```python
from build123d import *

# Parameters (mm, degrees)
F0_W     = 3.848
F0_H     = 8
F0_R     = 6
F0_R_2   = 4.05
F1_DEPTH = 5
F2_DEPTH = 3
F3_DEPTH = 50
F4_R     = 1


with BuildPart() as f1:
    # F0 (on Top) → F1 (new body)
    with BuildSketch(Plane.XY):
        with BuildLine():
            ThreePointArc((-8.75, 9.683053), (-3.977029, 7.706024), (-2, 2.933053))
            ThreePointArc((-2, 2.933053), (-3.977029, -1.839918), (-8.75, -3.816947))
            Line((-8.75, -3.816947), (8.75, -3.816947))
            ThreePointArc((8.75, -3.816947), (2, 2.933053), (8.75, 9.683053))
            Line((8.75, 9.683053), (-8.75, 9.683053))
        make_face()
        with Locations((0, 2.933053)):
            Rectangle(F0_W, F0_H, mode=Mode.SUBTRACT)
        with BuildLine():
            ThreePointArc((-8.75, -3.816947), (-3.977029, -1.839918), (-2, 2.933053))
            ThreePointArc((-2, 2.933053), (-3.977029, 7.706024), (-8.75, 9.683053))
            ThreePointArc((-8.75, 9.683053), (-15.5, 2.933053), (-8.75, -3.816947))
        make_face()
        with Locations((-8.75, 2.933053)):
            Circle(F0_R, mode=Mode.SUBTRACT)
        with BuildLine():
            ThreePointArc((15.5, 2.933053), (13.522971, 7.706024), (8.75, 9.683053))
            ThreePointArc((8.75, 9.683053), (2, 2.933053), (8.75, -3.816947))
            ThreePointArc((8.75, -3.816947), (13.522971, -1.839918), (15.5, 2.933053))
        make_face()
        with Locations((8.75, 2.933053)):
            Circle(F0_R, mode=Mode.SUBTRACT)
        with Locations((-8.75, 2.933053)):
            Circle(F0_R)
        with Locations((-8.75, 2.933053)):
            Circle(F0_R_2, mode=Mode.SUBTRACT)
        with Locations((8.75, 2.933053)):
            Circle(F0_R)
        with Locations((8.75, 2.933053)):
            Circle(F0_R_2, mode=Mode.SUBTRACT)
    extrude(amount=F1_DEPTH)

    # F0 (on Top) → F2 (cut)
    with BuildSketch(Plane.XY):
        with Locations((-8.75, 2.933053)):
            Circle(F0_R)
        with Locations((-8.75, 2.933053)):
            Circle(F0_R_2, mode=Mode.SUBTRACT)
        with Locations((8.75, 2.933053)):
            Circle(F0_R)
        with Locations((8.75, 2.933053)):
            Circle(F0_R_2, mode=Mode.SUBTRACT)
    extrude(amount=F2_DEPTH, mode=Mode.SUBTRACT)

    # F0 (on Top) → F3 (join)
    with BuildSketch(Plane.XY):
        with Locations((0, 2.933053)):
            Rectangle(F0_W, F0_H)
    extrude(amount=F3_DEPTH)

    # F4
    f4_edges = [f1.edges().sort_by_distance(p)[0] for p in [
        (-1.924, -1.066947, 27.5),
        (1.924, -1.066947, 27.5),
        (1.924, 6.933053, 27.5),
        (-1.924, 6.933053, 27.5),
    ]]
    fillet(f4_edges, radius=F4_R)


solid = f1.part
```
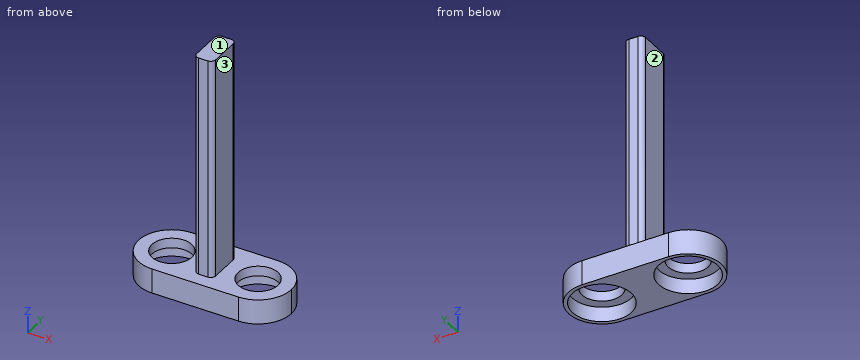
Read the model definition and answer for the solid it produces. Units are mm, in the model's axes. Face numbers are marked on the shaded views. A direction names the side the tool comes from. Give positions to 0.01 mm unless a question says otherwise; leave off trailing zeros. Write each loop counter-clockwise with the first axis right and the second up, starting at its lowest first coordinate (ties: lowest second). Pieces come first, ordered by that corner, then holes. Notation, with made-up numbers: (28, 6) -> (50, 6) arc R12 ccw to (50, 21) -> close; hole circle Ø4 at (42, 47.25). An arc over 180 degrees is marked (long way). Answer as a JSON object with one key per item and string values.
1) Section B-B on x = -6.5 is taken. Write down the section's boundary in (y, z).
Findings below:
{"outline": "(-3.82, 0) -> (-2.63, 0) -> (-2.63, 3) -> (-0.43, 3) -> (-0.43, 5) -> (-3.82, 5) -> close; (6.3, 3) -> (8.5, 3) -> (8.5, 0) -> (9.68, 0) -> (9.68, 5) -> (6.3, 5) -> close"}
2) A tool of negligible diameter and unlimited length cuts with its end or side. For the marked faces 1, 2 and 3, from which of +Z, -Z, +X, -X, +Y, -Y can it reach the whole face along a straight path? Write none if from no direction.
Findings below:
{"face 1": "+Z, +X, -X, +Y, -Y", "face 2": "+Z, -X, +Y, -Y", "face 3": "+Z, +X, +Y, -Y"}
3) Section D-D on y = 0.5 is taken. Write down the section's boundary in (x, z).
Findings below:
{"outline": "(-15.05, 0) -> (-14.23, 0) -> (-14.23, 3) -> (-11.99, 3) -> (-11.99, 5) -> (-15.05, 5) -> close; (-5.51, 3) -> (-3.27, 3) -> (-3.27, 0) -> (3.27, 0) -> (3.27, 3) -> (5.51, 3) -> (5.51, 5) -> (1.92, 5) -> (1.92, 50) -> (-1.92, 50) -> (-1.92, 5) -> (-5.51, 5) -> close; (11.99, 3) -> (14.23, 3) -> (14.23, 0) -> (15.05, 0) -> (15.05, 5) -> (11.99, 5) -> close"}
4) Straight lines are drawn through the part: probe 1 along Y at (x, z) = (-8.75, 0.8); probe 2 along Y at (x, z) = (9, 3.5); probe 3 along Z at (x, y) = (-4, 9). For each, find the intervals that lie inside material, in ascending order. Write a range as from..to.
Findings below:
{"probe 1": "y = -3.82..-3.07, 8.93..9.68", "probe 2": "y = -3.81..-1.11, 6.98..9.68", "probe 3": "z = 0..5"}
5) Section C-C on z = 37.5 is taken. Write down the section's boundary in (x, y).
Findings below:
{"outline": "(-1.92, -0.07) arc R1 ccw to (-0.92, -1.07) -> (0.92, -1.07) arc R1 ccw to (1.92, -0.07) -> (1.92, 5.93) arc R1 ccw to (0.92, 6.93) -> (-0.92, 6.93) arc R1 ccw to (-1.92, 5.93) -> close"}
6) Section A-A on y = 5 is taken. Write down the section's boundary in (x, z).
Findings below:
{"outline": "(-15.18, 0) -> (-14.38, 0) -> (-14.38, 3) -> (-12.23, 3) -> (-12.23, 5) -> (-15.18, 5) -> close; (-5.27, 3) -> (-3.12, 3) -> (-3.12, 0) -> (3.12, 0) -> (3.12, 3) -> (5.27, 3) -> (5.27, 5) -> (1.92, 5) -> (1.92, 50) -> (-1.92, 50) -> (-1.92, 5) -> (-5.27, 5) -> close; (12.23, 3) -> (14.38, 3) -> (14.38, 0) -> (15.18, 0) -> (15.18, 5) -> (12.23, 5) -> close"}
7) Flat-ended cylindrical pins translate along their axes: pin 1 Ø5 at (x, z) = (-3.5, 28.5) entering from +Y; pin 2 Ø4 at (x, y) = (5.5, 5.5) entering from +Z; pin 3 Ø3 at (y, z) = (4, 18.5) entering from -X. Find the tip coordinate at first contact, or state that the pin passes through.
Findings below:
{"pin 1": "stops at y = 6.93", "pin 2": "stops at z = 5", "pin 3": "stops at x = -1.92"}
